Part model, mm, in its own coordinate system. A direction names the side the tool comes from. Give positions to 0.01 mm unless a question says otherwise; leave off trailing zeros. Write each loop counter-clockwise with the first axis right and the second up, starting at its lowest first coordinate (ties: lowest second). Pieces come first, ordered by that corner, then holes.
from build123d import *

# Parameters (mm, degrees)
SKETCH1_W           = 90
SKETCH1_H           = 90
BOSS_EXTRUDE1_DEPTH = 60
SKETCH2_R           = 45
BOSS_EXTRUDE2_DEPTH = 170
SKETCH3_R           = 17
BOSS_EXTRUDE3_DEPTH = 5
SKETCH4_R           = 7.5
BOSS_EXTRUDE4_DEPTH = 33.5
CUT_EXTRUDE1_REACH  = 240.642
SKETCH5_R           = 3.5
FILLET1_R           = 7
CUT_EXTRUDE2_START  = -25
SKETCH6_R           = 45
SKETCH6_R_2         = 43
CUT_EXTRUDE2_DEPTH  = 25


with BuildPart() as part:
    # Sketch1 → Boss-Extrude1 (new body)
    with BuildSketch(Plane.XY):
        Rectangle(SKETCH1_W, SKETCH1_H)
    extrude(amount=BOSS_EXTRUDE1_DEPTH)

    # Sketch2 → Boss-Extrude2 (add)
    with BuildSketch(Plane(origin=(0, 0, 0), x_dir=(-1, 0, 0), z_dir=(0, 0, -1))):
        Circle(SKETCH2_R)
    extrude(amount=BOSS_EXTRUDE2_DEPTH)

    # Sketch3 → Boss-Extrude3 (add)
    with BuildSketch(Plane.XY.offset(60)):
        with Locations((0, 18)):
            Circle(SKETCH3_R)
    extrude(amount=BOSS_EXTRUDE3_DEPTH)

    # Sketch4 → Boss-Extrude4 (add)
    with BuildSketch(Plane.XY.offset(65)):
        with Locations((0, 18)):
            Circle(SKETCH4_R)
    extrude(amount=BOSS_EXTRUDE4_DEPTH)

    # Sketch5 → Cut-Extrude1 (cut, up to next)
    with BuildSketch(Plane.XY.offset(60), mode=Mode.PRIVATE) as cut_extrude1_sk1:
        with Locations((-37, 37)):
            Circle(SKETCH5_R)
    cut_extrude1_tool1 = extrude(cut_extrude1_sk1.sketch, amount=-CUT_EXTRUDE1_REACH, mode=Mode.PRIVATE) & part.part
    # Sketch5 → Cut-Extrude1 (cut, up to next)
    with BuildSketch(Plane.XY.offset(60), mode=Mode.PRIVATE) as cut_extrude1_sk2:
        with Locations((37, 37)):
            Circle(SKETCH5_R)
    cut_extrude1_tool2 = extrude(cut_extrude1_sk2.sketch, amount=-CUT_EXTRUDE1_REACH, mode=Mode.PRIVATE) & part.part
    # Sketch5 → Cut-Extrude1 (cut, up to next)
    with BuildSketch(Plane.XY.offset(60), mode=Mode.PRIVATE) as cut_extrude1_sk3:
        with Locations((37, -37)):
            Circle(SKETCH5_R)
    cut_extrude1_tool3 = extrude(cut_extrude1_sk3.sketch, amount=-CUT_EXTRUDE1_REACH, mode=Mode.PRIVATE) & part.part
    # Sketch5 → Cut-Extrude1 (cut, up to next)
    with BuildSketch(Plane.XY.offset(60), mode=Mode.PRIVATE) as cut_extrude1_sk4:
        with Locations((-37, -37)):
            Circle(SKETCH5_R)
    cut_extrude1_tool4 = extrude(cut_extrude1_sk4.sketch, amount=-CUT_EXTRUDE1_REACH, mode=Mode.PRIVATE) & part.part
    add(cut_extrude1_tool1.solids().sort_by_distance((-37, 37, 60))[0], mode=Mode.SUBTRACT)
    add(cut_extrude1_tool2.solids().sort_by_distance((37, 37, 60))[0], mode=Mode.SUBTRACT)
    add(cut_extrude1_tool3.solids().sort_by_distance((37, -37, 60))[0], mode=Mode.SUBTRACT)
    add(cut_extrude1_tool4.solids().sort_by_distance((-37, -37, 60))[0], mode=Mode.SUBTRACT)

    # Fillet1
    fillet1_edges = [part.edges().sort_by_distance(p)[0] for p in [
        (45, -45, 30),
        (-45, -45, 30),
        (-45, 45, 30),
        (45, 45, 30),
    ]]
    fillet(fillet1_edges, radius=FILLET1_R)

    # Sketch6 → Cut-Extrude2 (cut)
    with BuildSketch(Plane(origin=(0, 0, -170), x_dir=(-1, 0, 0), z_dir=(0, 0, -1)).offset(CUT_EXTRUDE2_START)):
        Circle(SKETCH6_R)
        Circle(SKETCH6_R_2, mode=Mode.SUBTRACT)
    extrude(amount=CUT_EXTRUDE2_DEPTH, mode=Mode.SUBTRACT)


solid = part.part
1) Saw through at C-C (z = -45). Write the cut outline in (x, y).
Check result:
outline: circle Ø90 at (0, 0)
2) Mould opens along Y. For faces 6 (the cylindrical face through (42.9, 43, 30.4)), 7 (the cylindrical face through (34.42, -34.635, 30.42)), 8 (the cylindrical face through (-20.765, -39.923, -71.485)) say: +Y half, -Y half, draft (parallel to the pull), parting line (faces both ways), or undercut.
Check result:
face 6: +Y half
face 7: undercut
face 8: parting line
3) Saw through at D-D (y = -8). Write the cut outline in (x, z).
Check result:
outline: (-45, 0) - (-44.28, 0) - (-44.28, -145) - (-42.25, -145) - (-42.25, -170) - (42.25, -170) - (42.25, -145) - (44.28, -145) - (44.28, 0) - (45, 0) - (45, 60) - (-45, 60) - close
4) Drill centre lines: L1, parallel to Y at x = -37, z = 46.5; L2, parallel to Z at x = 38.5, y = 24; L3, parallel to Z at x = -2.5, y = 0. Where is each one in solid material? Low to high.
Check result:
L1: y = -45 to -40.5, -33.5 to 33.5, 40.5 to 45
L2: z = 0 to 60
L3: z = -170 to 60
5) 3-axis set-ups, long thin cutter, end or side, ignore diameter. For faces 1 (the flat face through (-34, -34, 0)), 2 (the cylindrical face through (34.42, 39.365, 30.42)), 3 (the cylindrical face through (5.598, 42.634, -157.325)), 4 (the flat face through (7, 14, 65)), 5 (the flat face through (34, 33, 0)): which of +Z, -Z, +X, -X, +Y, -Y reach the whole face in a straight line?
Check result:
face 1: -Z, -X, -Y
face 2: +Z, -Z
face 3: -Z
face 4: +Z
face 5: -Z, +X, +Y
6) Flat gauge pins, fed straight in: P1, Ø8, axis at x = -2, z = -102, coming from the +Y side; P2, Ø3, axis at y = 34.5, z = -34, coming from the -X side; P3, Ø12, axis at y = 33.5, z = 66.5, coming from the -X side; P4, Ø4, axis at x = 37, y = -37, coming from the +Z side. Where does each tip first touch, or does it go through?
Check result:
P1: stops at y = 45
P2: stops at x = -30.59
P3: stops at x = -13.97
P4: passes through
7) Saw through at B-B (y = 4.5). Write the cut outline in (x, z), and give its area (3 significant figures).
Check result:
outline: (-45, 0) - (-44.77, 0) - (-44.77, -145) - (-42.76, -145) - (-42.76, -170) - (42.76, -170) - (42.76, -145) - (44.77, -145) - (44.77, 0) - (45, 0) - (45, 60) - (10.33, 60) - (10.33, 65) - (-10.33, 65) - (-10.33, 60) - (-45, 60) - close
area: 20,600 mm2
8) Saw through at A-A (x = 25.5). Write the cut outline in (y, z).
Check result:
outline: (-45, 0) - (-37.08, 0) - (-37.08, -145) - (-34.62, -145) - (-34.62, -170) - (34.62, -170) - (34.62, -145) - (37.08, -145) - (37.08, 0) - (45, 0) - (45, 60) - (-45, 60) - close
